The model under review builds one solid part; all positions refer to its coordinate system, in mm. A direction names the side the tool comes from. Round coordinates to 2 decimals unless told otherwise and drop trailing zeros. Order: outer loops, then holes, each group sorted by start corner. A loop starts at its lowest first (then second) coordinate and runs counter-clockwise, first axis right, second up. Notation, with made-up numbers: (-23, -28) -> (11, -28) arc R14 cw to (11, -20) -> close; hole circle Ø8 at (35.25, -2). An arc over 180 degrees is marked (long way). Use a Markdown table: item, result. Add a question column.
```python
from build123d import *

# Parameters (mm, degrees)
F0_W         = 25
F0_H         = 44
F1_DEPTH     = 60
F0_W_2       = 50
F0_H_2       = 20
F0_R         = 2.5
F2_DEPTH     = 6
F3_R         = 8
F4_DEPTH     = 20
F5_R         = 2.5
F6_DEPTH     = 60
F7_W         = 14
F7_H         = 30
F8_DEPTH     = 20
F9_START     = 25
F2_FACE_R    = 2.5
F9_DEPTH     = 5
F10_T1_DEPTH = 114.544511501
F10_T3_DEPTH = 115.544511501
F10_T5_DEPTH = 116
F10_T7_DEPTH = 115
F11_R        = 2.75
F12_DEPTH    = 32
F13_W        = 50
F13_H        = 18.5
F14_DEPTH    = 54
F16_DEPTH    = 18.5
F17_R        = 12.5
F18_DEPTH    = 16.8
F19_R        = 7
F20_DEPTH    = 18.5
F21_R        = 7
F21_R_2      = 3
F21_R_3      = 5
F22_DEPTH    = 18.5
F23_T1_DEPTH = 24.6515369414


# Not quite as in the source:
# - a fillet or chamfer that OpenCascade refuses, or shapes differently, is made with other operations: its cross-section is extruded or revolved along the edge and cut away or added


with BuildPart() as f1:
    # F0 (on Top) → F1 (new body)
    with BuildSketch(Plane.XY):
        with Locations((37.5, 0)):
            Rectangle(F0_W, F0_H)
    extrude(amount=F1_DEPTH)

    # F0 (on Top) → F2 (join)
    with BuildSketch(Plane.XY):
        with Locations((0, 32)):
            Rectangle(F0_W_2, F0_H_2)
        with Locations((0, 34.5)):
            Circle(F0_R, mode=Mode.SUBTRACT)
        Rectangle(F0_W_2, F0_H)
        with Locations((0, -32)):
            Rectangle(F0_W_2, F0_H_2)
        with Locations((0, -34.5)):
            Circle(F0_R, mode=Mode.SUBTRACT)
    extrude(amount=F2_DEPTH)

    # F3 (on face) → F4 (cut)
    with BuildSketch(Plane.YZ.offset(50)):
        Circle(F3_R)
        with Locations((0, 60)):
            Circle(F3_R)
    extrude(amount=-F4_DEPTH, mode=Mode.SUBTRACT)

    # F5 (on face) → F6 (cut)
    with BuildSketch(Plane.XY.offset(60)):
        with Locations((40, 15)):
            Circle(F5_R)
        with Locations((40, -15)):
            Circle(F5_R)
    extrude(amount=-F6_DEPTH, mode=Mode.SUBTRACT)

    # F7 (on face) → F8 (cut)
    with BuildSketch(Plane.YZ.offset(50)):
        with Locations((-15, 30)):
            Rectangle(F7_W, F7_H)
        with Locations((15, 30)):
            Rectangle(F7_W, F7_H)
    extrude(amount=-F8_DEPTH, mode=Mode.SUBTRACT)

    # F2_face (on face) → F9 (join)
    with BuildSketch(Plane.XY.offset(6).offset(F9_START)):
        Polygon((-25, 42), (-25, -42), (25, -42), (25, -22), (25, 22), (25, 42), align=None)
        with Locations((0, 34.5)):
            Circle(F2_FACE_R, mode=Mode.SUBTRACT)
        with Locations((0, -34.5)):
            Circle(F2_FACE_R, mode=Mode.SUBTRACT)
    extrude(amount=F9_DEPTH)

    # F10: fillet of radius 22 on 8 edges, made by hand

    # F10_s2 → F10_t1 (cut)
    with BuildSketch(Plane.XY.offset(-23.7722557505)):
        with BuildLine():
            ThreePointArc((25, -22), (17.923494674, -36.2480768093), (3.0910976998, -42))
            Line((3.0910976998, -42), (25, -42))
            Line((25, -42), (25, -22))
        make_face()
        with BuildLine():
            ThreePointArc((25, 22), (17.923494674, 36.2480768093), (3.0910976998, 42))
            Line((3.0910976998, 42), (25, 42))
            Line((25, 42), (25, 22))
        make_face()
    extrude(amount=F10_T1_DEPTH, mode=Mode.SUBTRACT)

    # F10_s4 → F10_t3 (cut)
    with BuildSketch(Plane.XY.offset(-54.7722557505)):
        with BuildLine():
            ThreePointArc((3.0910976998, -42), (17.923494674, -36.2480768093), (25, -22))
            Line((25, -22), (25, -42))
            Line((25, -42), (3.0910976998, -42))
        make_face()
        with BuildLine():
            ThreePointArc((25, 22), (17.923494674, 36.2480768093), (3.0910976998, 42))
            Line((3.0910976998, 42), (25, 42))
            Line((25, 42), (25, 22))
        make_face()
    extrude(amount=F10_T3_DEPTH, mode=Mode.SUBTRACT)

    # F10_s6 → F10_t5 (cut)
    with BuildSketch(Plane.XY.offset(-55)):
        with BuildLine():
            ThreePointArc((-25, -20), (-18.5563491861, -35.5563491861), (-3, -42))
            Line((-3, -42), (-25, -42))
            Line((-25, -42), (-25, -20))
        make_face()
        with BuildLine():
            ThreePointArc((-3, 42), (-18.5563491861, 35.5563491861), (-25, 20))
            Line((-25, 20), (-25, 42))
            Line((-25, 42), (-3, 42))
        make_face()
    extrude(amount=F10_T5_DEPTH, mode=Mode.SUBTRACT)

    # F10_s8 → F10_t7 (cut)
    with BuildSketch(Plane.XY.offset(-24)):
        with BuildLine():
            ThreePointArc((-25, -20), (-18.5563491861, -35.5563491861), (-3, -42))
            Line((-3, -42), (-25, -42))
            Line((-25, -42), (-25, -20))
        make_face()
        with BuildLine():
            ThreePointArc((-3, 42), (-18.5563491861, 35.5563491861), (-25, 20))
            Line((-25, 20), (-25, 42))
            Line((-25, 42), (-3, 42))
        make_face()
    extrude(amount=F10_T7_DEPTH, mode=Mode.SUBTRACT)

    # F11 (on face) → F12 (cut)
    with BuildSketch(Plane.XY.offset(36)):
        with Locations((18, 17)):
            Circle(F11_R)
        with Locations((-18, 17)):
            Circle(F11_R)
        with Locations((-18, -17)):
            Circle(F11_R)
        with Locations((18, -17)):
            Circle(F11_R)
    extrude(amount=-F12_DEPTH, mode=Mode.SUBTRACT)

    # F13 (on face) → F14 (join)
    with BuildSketch(Plane.XY.offset(6)):
        Rectangle(F13_W, F13_H)
    extrude(amount=F14_DEPTH)

    # F15 (on face) → F16 (cut)
    with BuildSketch(Plane.XZ.offset(9.25)):
        Polygon((-25, 36), (25, 60), (-25, 60), align=None)
    extrude(amount=-F16_DEPTH, mode=Mode.SUBTRACT)

    # F17 (on face) → F18 (cut)
    with BuildSketch(Plane.XZ.offset(8)):
        with Locations((50, 30)):
            Circle(F17_R)
    extrude(amount=-F18_DEPTH, mode=Mode.SUBTRACT)

    # F19 (on face) → F20 (cut)
    with BuildSketch(Plane.XZ.offset(9.25)):
        with Locations((0, 18.5)):
            Circle(F19_R)
        with Locations((16, 18.5)):
            Circle(F19_R)
        with Locations((-16, 18.5)):
            Circle(F19_R)
    extrude(amount=-F20_DEPTH, mode=Mode.SUBTRACT)

    # F21 (on face) → F22 (cut)
    with BuildSketch(Plane.XZ.offset(9.25)):
        with Locations((16, 44)):
            Circle(F21_R)
        with Locations((-7.6543654317, 40)):
            Circle(F21_R_2)
        with Locations((2.1435935394, 42)):
            Circle(F21_R_3)
    extrude(amount=-F22_DEPTH, mode=Mode.SUBTRACT)

    # F23: chamfer of 2 on 4 edges, made by hand

    # F23_s2 → F23_t1 (cut)
    with BuildSketch(Plane.YZ.offset(30)):
        with BuildLine():
            Line((9.7979589711, 60), (7.8383671769, 58.4))
            ThreePointArc((7.8383671769, 58.4), (7.9565711479, 59.1675484588), (8, 60))
            Line((8, 60), (9.7979589711, 60))
        make_face()
        with BuildLine():
            Line((-9.7979589711, 60), (-7.8383671769, 58.4))
            ThreePointArc((-7.8383671769, 58.4), (-7.9565711479, 59.1675484588), (-8, 60))
            Line((-8, 60), (-9.7979589711, 60))
        make_face()
        with BuildLine():
            Line((9.7979589711, 0), (7.8383671769, 1.6))
            ThreePointArc((7.8383671769, 1.6), (7.9565711479, 0.8324515412), (8, 0))
            Line((8, 0), (9.7979589711, 0))
        make_face()
        with BuildLine():
            Line((-9.7979589711, 0), (-7.8383671769, 1.6))
            ThreePointArc((-7.8383671769, 1.6), (-7.9565711479, 0.8324515412), (-8, 0))
            Line((-8, 0), (-9.7979589711, 0))
        make_face()
    extrude(amount=F23_T1_DEPTH, mode=Mode.SUBTRACT)


solid = f1.part
```
Q1. Add section A-A (y = 11). Write out the cut boundary in (x, z), then the cut area to 3 significant figures.
Q2. Add section D-D (y = -27.5). Write out the cut boundary in (x, z), then the cut area to 3 significant figures.
Q3. Wall thickness on line 1 (Y direction, x = 40, z = 51); line 2 (Y direction, x = 0, z = 3.5); line 3 (Z direction, x = -5.5, y = -19): over which ranges is each line inside the solid? List them lowest first. Write a range as [from, to].
Q4. Machinability: for faces 1 (the cylindrical face through (-20.747, 17.121, 33.535)), 2 (the flat face through (42.4, 16.5, 15)), 3 (the flat face through (39.86, -8.83, 59.21)), which of the approach directions +Z, -Z, +X, -X, +Y, -Y give a long, thin tool a straight path to every point of the face, cutting with its end or side? Answer none if there is none.
Q5. Insertion check: pin 1 (8 mm diameter, centred on x = 30, z = 24, fed in from -Y); pin 2 (6 mm diameter, centred on x = 37.5, z = 28.5, fed in from -Y); pin 3 (5 mm diameter, centred on x = 18, y = -17, fed in from -Z); pin 4 (16.5 mm diameter, centred on x = -0.5, y = 33, fed in from +Z). Each pin has a flat end and moves straight along its axis. Give the tip position at first contact, or say it passes through.
Q6. Add section C-C (y = 1). Write out the cut boundary in (x, z).
Q7. Mouldability with a two-part tool opening along Z and no side actions: class faces 4 (the flat face through (-18, -17, 4)), 5 (the flat face through (38, -17, 45)), 6 (the cylindrical face through (18.091, 36.094, 33.465)) as pulls with the +Z half, pulls with the -Z half, needs draft (parallel to the pull), parting line crosses it, or undercut.
Q8. Add section B-B (x = -13.5). Write out the cut boundary in (y, z), then the cut area to 3 significant figures.
Report:
| question | item | result |
|---|---|---|
| 1 | outline | (-25, 0) -> (50, 0) -> (50, 15) -> (30, 15) -> (30, 45) -> (50, 45) -> (50, 60) -> (25, 60) -> (25, 36) -> (-25, 36) -> (-25, 31) -> (25, 31) -> (25, 6) -> (-25, 6) -> close |
| 1 | area | 1,450 mm² |
| 2 | outline | (-23.68, 0) -> (23.77, 0) -> (23.77, 6) -> (-23.68, 6) -> close; (-23.68, 31) -> (23.77, 31) -> (23.77, 36) -> (-23.68, 36) -> close |
| 2 | area | 522 mm² |
| 3 | line 1 | y = [-22, -17.5], [-12.5, 12.5], [17.5, 22] |
| 3 | line 2 | y = [-42, -37], [-32, 32], [37, 42] |
| 3 | line 3 | z = [0, 6], [31, 36] |
| 4 | face 1 | +Z |
| 4 | face 2 | +X, +Y |
| 4 | face 3 | +Z, +X |
| 5 | pin 1 | stops at y = -22 |
| 5 | pin 2 | stops at y = -8 |
| 5 | pin 3 | stops at z = 0 |
| 5 | pin 4 | stops at z = 36 |
| 6 | outline | (-25, 0) -> (30, 0) -> (30, 7.94) -> (50, 7.94) -> (50, 17.5) arc R12.5 cw to (50, 42.5) -> (50, 52.06) -> (30, 52.06) -> (30, 60) -> (25, 60) -> (-25, 36) -> close; hole circle Ø14 at (-16, 18.5); hole circle Ø6 at (-7.65, 40); hole circle Ø14 at (0, 18.5); hole circle Ø10 at (2.14, 42); hole circle Ø14 at (16, 18.5); hole circle Ø14 at (16, 44) |
| 7 | face 4 | pulls with the +Z half |
| 7 | face 5 | undercut |
| 7 | face 6 | needs draft |
| 8 | outline | (-39.33, 0) -> (39.33, 0) -> (39.33, 6) -> (9.25, 6) -> (9.25, 11.96) -> (-9.25, 11.96) -> (-9.25, 6) -> (-39.33, 6) -> close; (-39.33, 31) -> (-9.25, 31) -> (-9.25, 25.04) -> (9.25, 25.04) -> (9.25, 31) -> (39.33, 31) -> (39.33, 36) -> (9.25, 36) -> (9.25, 41.52) -> (-9.25, 41.52) -> (-9.25, 36) -> (-39.33, 36) -> close |
| 8 | area | 1,190 mm² |
